Could you check a few things on this model? Use its own coordinates, in mm. Face numbers are marked on the shaded views. A direction names the side the tool comes from. Round coordinates to 2 decimals unless told otherwise and drop trailing zeros. Loops run counter-clockwise (first coordinate to the right, second up) from the corner with the lowest first, then second, coordinate; pieces in that order, holes last. Notation, with made-up numbers: (67.25, 73) - (76.25, 73) arc R27 cw to (76.25, 109) - close; hole circle Ø5 at (47, 52.5). An arc over 180 degrees is marked (long way). Use one line per item in the form item = value.
```python
from build123d import *

# Parameters (mm, degrees)
F2_R = 5.08
F3_R = 3.048


with BuildPart() as f1:
    # F0 (on Front) → F1 (revolve)
    with BuildSketch(Plane.XZ):
        Polygon((0, -34.125851), (0, 67.474149), (-25.4, 67.474149), (-25.4, 29.374149), (-7.9375, 29.374149), (-7.9375, -21.425851), (-15.875, -21.425851), (-15.875, -34.125851), align=None)
    revolve(axis=Axis((0, 0, 9.330612), (0, 0, -1)))

    # F2
    f2_edges = [f1.edges().sort_by_distance(p)[0] for p in [
        (7.9375, 0, 29.374149),
        (15.875, 0, -21.425851),
    ]]
    fillet(f2_edges, radius=F2_R)

    # F3
    f3_edges = [f1.edges().sort_by_distance(p)[0] for p in [
        (25.4, 0, 29.374149),
    ]]
    fillet(f3_edges, radius=F3_R)


solid = f1.part
```
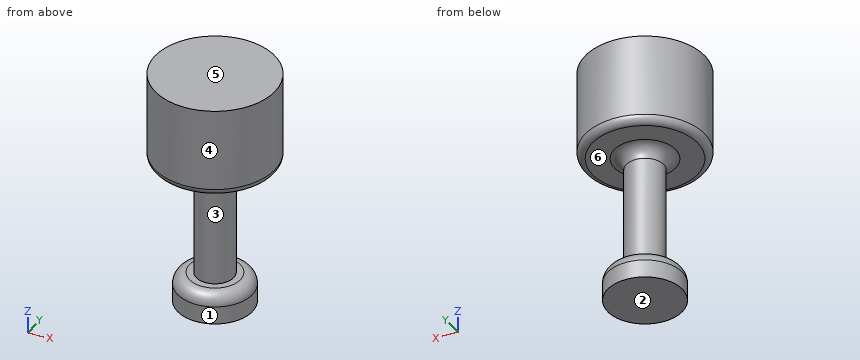
1. On a 3-axis mill with a long thin cutter (end or side, diameter ignored), from which of +Z, -Z, +X, -X, +Y, -Y can I reach the whole of each face in a straight line? I mean the marked faces 1, 2 and 3. Say none if no direction works.
Solution:
face_1 = -Z
face_2 = -Z, +X, -X, +Y, -Y
face_3 = none
2. Please list where these lines run through material, in increasing order: line 1 along Z through (x, y) = (7, 21.5); line 2 along X through (y, z) = (-23, 55); line 3 along X through (y, z) = (6.5, 44).
Solution:
line_1 = 29.39 to 67.47
line_2 = -10.78 to 10.78
line_3 = -24.55 to 24.55
3. If we section it at D-D, the plane z = 34: Write out the boundary of the cut face in (x, y), plus the area to 3 significant figures.
Solution:
outline = circle Ø50.8 at (0, 0)
area = 2,030 mm^2
4. We'd pull the mould along Z, two halves only. Please class the marked faces 4, 5 and 6: +Z half, -Z half, draft (parallel to the pull), parting line (faces both ways), or undercut.
Solution:
face_4 = draft
face_5 = +Z half
face_6 = undercut
5. If we section it at C-C, the plane z = -20: Write out the boundary of the cut face in (x, y) (1 decimal).
Solution:
outline = circle Ø15.9 at (0, 0)
6. If we section it at A-A, the plane x = 0: Write out the boundary of the cut face in (y, z) (1 decimal).
Solution:
outline = (-25.4, 32.4) arc R3 ccw to (-22.4, 29.4) - (-13, 29.4) arc R5.1 cw to (-7.9, 24.3) - (-7.9, -21.4) - (-10.8, -21.4) arc R5.1 ccw to (-15.9, -26.5) - (-15.9, -34.1) - (15.9, -34.1) - (15.9, -26.5) arc R5.1 ccw to (10.8, -21.4) - (7.9, -21.4) - (7.9, 24.3) arc R5.1 cw to (13, 29.4) - (22.4, 29.4) arc R3 ccw to (25.4, 32.4) - (25.4, 67.5) - (-25.4, 67.5) - close
7. For P1, Ø3, axis at y = -10, z = 6.5, coming from the +X side, with a flat end and sliding along its axis, tell me the tip position at first contact or that it passes through.
Solution:
P1 = through
